Geometry: final body of the model. Coordinates: model frame, mm. A direction names the side the tool comes from. Coordinates: 2 decimals unless noted, no trailing zeros. Answer as a JSON object with one key per item and string values. Group by question number.
Item 1: Set-up query: faces 1 (the flat face through (-34, 0, 8)), 2 (the cylindrical face through (-29.306, -6.219, 22.471)), 3 (the flat face through (37.4, -8, -0.2)). Return all of +Z, -Z, +X, -X, +Y, -Y with unobstructed straight access to the full face (end or side cutting, diameter ignored); none if empty.
Item 2: Line query: line 1 along Z through (x, y) = (0, -1.35); line 2 along Z through (x, y) = (7, -0.25). Output: solid intervals per line, ascending. Write a range as from..to.
Item 3: Mould query, pull axis Y, two halves, no side actions, for faces 4 (the cylindrical face through (35.04, -5.09, -11.04)), 5 (the flat face through (-11.4, 1.4, -34)), 6 (the conical face through (35.335, -7.84, -14.409)), 7 (the cylindrical face through (35.04, -2.29, -11.04)). Classes: pulls with the +Y half, pulls with the -Y half, needs draft (parallel to the pull), parting line crosses it, or undercut.
Item 4: First-contact query: pin 1 Ø4 at (x, y) = (18, -2.5) entering from -Z; pin 2 Ø5 at (y, z) = (-1, 26) entering from +X; pin 3 Ø4 at (y, z) = (-1.5, -9.5) entering from -X. Flat tips, straight axial feed; report the tip coordinate or a pass-through.
```python
from build123d import *

# Parameters (mm, degrees)
SKETCH_1_R               = 39
EXTRUDE_1_DEPTH          = 2
SKETCH_3_R               = 34.5
CUT_EXTRUDE_1_DEPTH      = 57.053545829
CUT_EXTRUDE_START        = -0.6
SKETCH_4_R               = 39
CUT_EXTRUDE_2_DEPTH      = 0.6
CHAMFER_1_SIZE           = 1.732
CHAMFER_1_SIZE2          = 0.999970666
CHAMFER_2_SIZE           = 1.2
CUT_REVOLVE_1_ANGLE      = 45
PATTERN_CIRCULAR_1_COUNT = 4
SKETCH_6_R               = 35.78
SKETCH_6_R_2             = 35.32
EXTRUDE_2_DEPTH          = 0.5


with BuildPart() as part:
    # 草图1 → 凸台-拉伸1 (new body)
    with BuildSketch(Plane(origin=(0, 0, 0), x_dir=(1, 0, 0), z_dir=(0, 1, 0))):
        with Locations(Location((0, 0, 0), (0, 0, 270))):
            Circle(SKETCH_1_R)
    extrude(amount=EXTRUDE_1_DEPTH)

    # 草图2 → 旋转1 (revolve)
    with BuildSketch(Plane(origin=(0, 0, 0), x_dir=(0.5000000000000016, 0, 0.8660254037844378), z_dir=(-0.8660254037844377, 0, 0.5000000000000014)), mode=Mode.PRIVATE) as revolve_1_sk:
        with BuildLine():
            Line((36.93, -8), (36.93, -7.5))
            Line((36.93, -7.5), (36.505, -7.075))
            Line((36.505, -7.075), (36.93, -6.65))
            Line((36.93, -6.65), (36.93, -5.8))
            Line((36.93, -5.8), (36.74, -5.61))
            Line((36.74, -5.61), (36.74, -4.59))
            Line((36.74, -4.59), (36.93, -4.4))
            Line((36.93, -4.4), (36.93, -3))
            Line((36.93, -3), (36.74, -2.81))
            Line((36.74, -2.81), (36.74, -1.79))
            Line((36.74, -1.79), (36.93, -1.6))
            Line((36.93, -1.6), (36.93, -1.4))
            ThreePointArc((36.93, -1.4), (36.519949494, -0.410050506), (35.53, 0))
            Line((35.53, 0), (39, 0))
            Line((39, 0), (39, -8))
            Line((39, -8), (36.93, -8))
        make_face()
    revolve(revolve_1_sk.sketch.rotate(Axis((0, 0, 0), (0, 1, 0)), 60), axis=Axis((0, 0, 0), (0, 1, 0)))

    # 草图3 → 切除-拉伸1 (cut, through all)
    with BuildSketch(Plane(origin=(0, 2, 0), x_dir=(1, 0, 0), z_dir=(0, 1, 0))):
        with Locations(Location((0, 0, 0), (0, 0, 270))):
            Circle(SKETCH_3_R)
    extrude(amount=-CUT_EXTRUDE_1_DEPTH, mode=Mode.SUBTRACT)

    # 草图4 → 切除-拉伸2 (cut)
    with BuildSketch(Plane(origin=(0, 2, 0), x_dir=(1, 0, 0), z_dir=(0, 1, 0)).offset(CUT_EXTRUDE_START)):
        Circle(SKETCH_4_R)
    extrude(amount=CUT_EXTRUDE_2_DEPTH, mode=Mode.SUBTRACT)

    # 倒角1
    chamfer_1_edges = [part.edges().sort_by_distance(p)[0] for p in [
        (0, 1.4, -39),
    ]]
    chamfer_1_side = [part.faces().sort_by_distance(p)[0] for p in [
        (-27.577164466, -3.3, -27.577164466),
    ]]
    chamfer(chamfer_1_edges, length=CHAMFER_1_SIZE, length2=CHAMFER_1_SIZE2, reference=chamfer_1_side[0])

    # 倒角2
    chamfer_2_edges = [part.edges().sort_by_distance(p)[0] for p in [
        (0, 1.4, -34.5),
    ]]
    chamfer(chamfer_2_edges, length=CHAMFER_2_SIZE)

    # 草图5 → 切除-旋转1 (revolve, cut)
    with BuildSketch(Plane.XY):
        Polygon((39, -8), (39, -7), (38, -8), align=None)
    cut_revolve_1 = revolve(axis=Axis((0, 0, 0), (0, 1, 0)), revolution_arc=CUT_REVOLVE_1_ANGLE, mode=Mode.SUBTRACT)

    # 阵列(圆周)1: 切除-旋转1 ×4 about axis
    pattern_circular_1_axis = Axis((0, 0, 0), (0, 1, 0))
    for i in range(1, PATTERN_CIRCULAR_1_COUNT):
        add(cut_revolve_1.rotate(pattern_circular_1_axis, i * 360 / PATTERN_CIRCULAR_1_COUNT), mode=Mode.SUBTRACT)

    # 草图6 → 凸台-拉伸2 (add)
    with BuildSketch(Plane.XZ):
        Circle(SKETCH_6_R)
        with Locations(Location((0, 0, 0), (0, 0, 270))):
            Circle(SKETCH_6_R_2, mode=Mode.SUBTRACT)
    extrude(amount=EXTRUDE_2_DEPTH)


solid = part.part
```
Checks:
{
 "1": {"face 1": "-Y", "face 2": "none", "face 3": "+Z, -Z, +X, -X, -Y"},
 "2": {"line 1": "-39..-36.93, 36.93..39", "line 2": "-38.32..-35.65, -35.09..-34.62, 34.62..35.09, 35.65..38.32"},
 "3": {"face 4": "undercut", "face 5": "pulls with the +Y half", "face 6": "pulls with the -Y half", "face 7": "undercut"},
 "4": {"pin 1": "z = -35.57", "pin 2": "x = 31.12", "pin 3": "x = -38.27"}
}
